Build history of the part. All positions in model axes, mm. A direction names the side the tool comes from. Round coordinates to 2 decimals unless told otherwise and drop trailing zeros. Order: outer loops, then holes, each group sorted by start corner. A loop starts at its lowest first (then second) coordinate and runs counter-clockwise, first axis right, second up. Notation, with made-up numbers: (54.5, 51.25) -> (103.5, 51.25) arc R22 cw to (103.5, 75.25) -> close; hole circle Ø5 at (6, 4.5). An arc over 180 degrees is marked (long way). Answer as a JSON object with one key per item and string values.
Autodesk Inventor part; units mm, degrees
ref_plane "XZ Plane" through (0, 0, 0) normal (0, 1, 0) x (-1, 0, 0)
ref_plane "XY Plane" through (0, 0, 0) normal (0, 0, 1) x (1, 0, 0)
sketch "Sketch1" plane through (0, 0, 0) normal (0, 0, 1) x (1, 0, 0)
  line L0 (-26.797, 31.75) -> (26.797, 31.75)
  line L1 (26.797, 31.75) -> (26.797, -31.75)
  line L2 (26.797, -31.75) -> (-26.797, -31.75)
  line L3 (-26.797, -31.75) -> (-26.797, 31.75)
  point P0 (0, 0)
  point P1 (-26.797, 0)
  point P2 (0, 31.75)
  dimension "d0" = 53.594
  dimension "d1" = 63.5
extrude "Extrusion1" add sketch "Sketch1" along normal blind 1.5875
sketch "Sketch9" plane through (0, 0, 1.5875) normal (0, 0, 1) x (1, 0, 0)
  line L0 (26.797, 31.75) -> (26.797, -31.75)
  line L1 (-26.797, -31.75) -> (-26.797, 31.75)
  line L2 (26.797, -31.75) -> (-26.797, -31.75)
  line L3 (-26.797, -31.75) -> (26.797, -31.75)
  line L4 (26.797, -31.75) -> (26.797, -40.7924)
  line L5 (26.797, -40.7924) -> (-26.797, -40.7924)
  line L6 (-26.797, -40.7924) -> (-26.797, -31.75)
  line L7 (-26.797, 31.75) -> (26.797, 31.75)
  point P0 (0, 0)
  dimension "d60" = 72.5424
extrude "Extrusion5" add sketch "Sketch9" against normal up to surface (1.5875 mm away) contours L4 L5 L6 L2
sketch "Sketch2" plane through (0, 0, 1.5875) normal (0, 0, 1) x (1, 0, 0)
  line L0 (-26.797, -39.1922) -> (26.797, -39.1922)
  line L1 (26.797, -40.7924) -> (-26.797, -40.7924)
  line L2 (26.797, -40.7924) -> (26.797, 31.75)
  line L3 (-26.797, -40.7924) -> (26.797, -40.7924)
  line L4 (-26.797, -40.7924) -> (-26.797, -39.1922)
  line L5 (26.797, -40.7924) -> (26.797, -39.1922)
  point P0 (-26.797, -31.75)
  point P1 (0, 0)
  dimension "d4" = 53.594
  dimension "d59" = 1.6002
extrude "Extrusion2" add sketch "Sketch2" along normal blind 12.7
sketch "Sketch6" plane through (0, 0, 1.5875) normal (0, 0, 1) x (1, 0, 0)
  line L0 (26.797, 31.75) -> (26.797, -29.3687)
  line L1 (-26.797, 31.75) -> (26.797, 31.75)
  line L2 (-26.797, -29.3687) -> (-26.797, 31.75)
  arc A0 (20.447, -21.844) -> (23.9286, -10.1836) centre (20.447, -15.494) ccw
  arc A1 (23.4121, -8.0836) -> (23.9286, -10.1836) centre (24.799, -8.856) ccw
  arc A2 (23.4121, -8.0836) -> (26.797, 4.953) centre (0, 4.953) ccw
  line L3 (26.797, 25.4) -> (26.797, 4.953)
  arc A3 (26.797, 25.4) -> (20.447, 31.75) centre (20.447, 25.4) ccw
  line L4 (14.199, 31.75) -> (20.447, 31.75)
  line L5 (-14.199, 31.75) -> (14.199, 31.75)
  line L6 (-20.447, 31.75) -> (-14.199, 31.75)
  arc A4 (-20.447, 31.75) -> (-26.797, 25.4) centre (-20.447, 25.4) ccw
  line L7 (-26.797, 4.953) -> (-26.797, 25.4)
  arc A5 (-26.797, 4.953) -> (-23.4121, -8.0836) centre (0, 4.953) ccw
  arc A6 (-23.9286, -10.1836) -> (-23.4121, -8.0836) centre (-24.799, -8.856) ccw
  arc A7 (-23.9286, -10.1836) -> (-20.447, -21.844) centre (-20.447, -15.494) ccw
  line L8 (20.447, -21.844) -> (-20.447, -21.844)
  arc A8 (-23.9286, -10.1836) -> (-26.797, -15.494) centre (-20.447, -15.494) ccw
  arc A9 (26.797, -15.494) -> (23.9286, -10.1836) centre (20.447, -15.494) ccw
  arc A10 (23.4121, -8.0836) -> (23.9286, -10.1836) centre (24.799, -8.856) ccw
  arc A11 (-23.9286, -10.1836) -> (-23.4121, -8.0836) centre (-24.799, -8.856) ccw
  point P0 (0, 0)
extrude "Extrusion4" cut sketch "Sketch6" against normal up to next contours L0 A3 L1 | L0 A0 A1 A2 | A4 L2 L1 | L2 A5 A6 A7
sketch "Sketch7" plane through (0, 0, 1.5875) normal (0, 0, 1) x (1, 0, 0)
  arc A0 (26.797, 25.4) -> (20.447, 31.75) centre (20.447, 25.4) ccw
  arc A1 (-20.447, 31.75) -> (-26.797, 25.4) centre (-20.447, 25.4) ccw
  arc A2 (-23.9286, -10.1836) -> (-26.797, -15.494) centre (-20.447, -15.494) ccw
  arc A3 (26.797, -15.494) -> (23.9286, -10.1836) centre (20.447, -15.494) ccw
  point P0 (0, 0)
hole "Hole3" at (-20.447, 25.4, 1.5875) at (20.447, 25.4, 1.5875) at (20.447, -15.494, 1.5875) at (-20.447, -15.494, 1.5875) direction (0, 0, -1) diameter 3.81 end through all
ref_plane "Work Plane1" through (-26.797, -30.1625, 2.3812) normal (0, 1, 0) x (1, 0, 0)
fillet "Fillet3" radius 1.6002 1 edges at (0, -39.1922, 1.5875)
fillet "Fillet4" radius 3.175 1 edges at (0, -40.7924, 0)
fillet "Fillet5" radius 3.175 2 edges at (-26.797, -39.9923, 14.2875) (26.797, -39.9923, 14.2875)
sketch "Sketch10" plane through (-26.797, -39.1922, 3.1877) normal (0, 1, 0) x (1, 0, 0)
  circle A0 centre (44.831, -5.4264) radius 2.4116
  point P0 (26.797, 3.1877)
hole "Hole6" at (18.034, -39.1922, 8.6141) direction (0, -1, 0) diameter 5.1054 end through all
mirror "Mirror1" about plane through (0, 0, 0) normal (1, 0, 0) of "Hole6"
properties part number "Pneumatics_VIAIR_0090_01" material "Aluminum-6061"
1) Probe L1, parallel to Z at x = 5.5, y = -32; L2, parallel to Y at x = 8, z = 3.5; L3, parallel to Y at x = 24, z = 1.5. List the from-to ranges inside material, lowest first. Write a range as from..to.
Checked values:
{"L1": "z = 0..1.59", "L2": "y = -40.79..-39.19", "L3": "y = -40.31..-10.23, -6.97..30.66"}
2) Cut at A-A, the plane z = 9.5. Give the cut face in (x, y), plus the area to 3 significant figures.
Checked values:
{"outline": "(-26.8, -40.79) -> (-20.43, -40.79) -> (-20.43, -39.19) -> (-26.8, -39.19) -> close; (-15.64, -40.79) -> (15.64, -40.79) -> (15.64, -39.19) -> (-15.64, -39.19) -> close; (20.43, -40.79) -> (26.8, -40.79) -> (26.8, -39.19) -> (20.43, -39.19) -> close", "area": "70.4 mm²"}
3) Which spindle directions (+Z, -Z, +X, -X, +Y, -Y) get a long thin tool onto all of the face, cutting with end or side? Do faces 1 (the face through (26.055, -12.515, 0.805)), 2 (the face through (-24.887, 29.939, 0.805)), 3 (the face through (-25.96, -1.69, 0.8)). Say none if no direction does.
Checked values:
{"face 1": "+Z, -Z, +X", "face 2": "+Z, -Z, -X, +Y", "face 3": "+Z, -Z, -X"}
4) Cut at C-C, the plane y = 10. Give the cut face in (x, z).
Checked values:
{"outline": "(-26.8, 0) -> (26.8, 0) -> (26.8, 1.59) -> (-26.8, 1.59) -> close"}
5) Pull direction Y, two halves, no side cores. Call faces 4 (the face through (-26.013, -12.438, 0.805)), 5 (the face through (25.842, -39.981, 13.382)), 6 (the face through (0.375, -38.736, 2.069)), 7 (the face through (0, -40.792, 9)): pulls with the +Y half, pulls with the -Y half, needs draft (parallel to the pull), parting line crosses it, or undercut.
Checked values:
{"face 4": "undercut", "face 5": "needs draft", "face 6": "pulls with the +Y half", "face 7": "pulls with the -Y half"}
6) Flat gauge pins, fed straight in: pin 1 Ø5 at (x, y) = (-20.447, -15.494) entering from +Z; pin 2 Ø2.5 at (x, y) = (-20.447, 25.4) entering from +Z; pin 3 Ø5 at (x, z) = (21, 10) entering from +Y. Where does each tip first touch, or does it go through?
Checked values:
{"pin 1": "stops at z = 1.59", "pin 2": "passes through", "pin 3": "stops at y = -39.19"}
7) Cut at D-D, the plane z = 4.25. Give the cut face in (x, y).
Checked values:
{"outline": "(-26.8, -40.79) -> (26.8, -40.79) -> (26.8, -39.19) -> (-26.8, -39.19) -> close"}
